Input: dimensioned drawing with shaded views. Units: mm. Origin: part minimum x, y, z. A direction names the side the tool comes from. Round coordinates to 2 decimals unless told otherwise and drop trailing zeros. Order: outer loops, then holes, each group sorted by start corner. A loop starts at its lowest first (then second) coordinate and runs counter-clockwise, first axis right, second up. Notation, with made-up numbers: M 75.5,74 L 80.5,74 A17 ccw 80.5,100 Z; hole C -10,42 d1. An arc over 180 degrees is marked long. Use one line per item in the form item = value. Start each with the question number.
Q1. Section A-A (y = 8). Return the cut outline in (x, z).
Q2. Contact query for flat-ended pins moving along their axis: pin 1 (8 mm diameter, centred on x = 2.5, y = 24, fed in from -Z); pin 2 (11 mm diameter, centred on y = 53, z = 24, fed in from +X); pin 3 (1 mm diameter, centred on x = 18.5, y = 42.5, fed in from +Z). Output: stop coordinate, or through.
Q3. Section D-D (y = 50). Return the cut outline in (x, z).
Q4. Material intervals for probe 1 along Y at (x, z) = (4.5, 20); probe 2 along Z at (x, y) = (14.25, 7.5), sorted ascending.
Q5. Reachability of the marked faces 1 and 2 from +Z, -Z, +X, -X, +Y, -Y: full face, straight path, thin tool, end or side. Return the list, or none.
Q6. Section B-B (x = 2.5). Return the cut outline in (y, z).
Q7. Section C-C (z = 24.5). Return the cut outline in (x, y), plus the area to 3 significant figures.
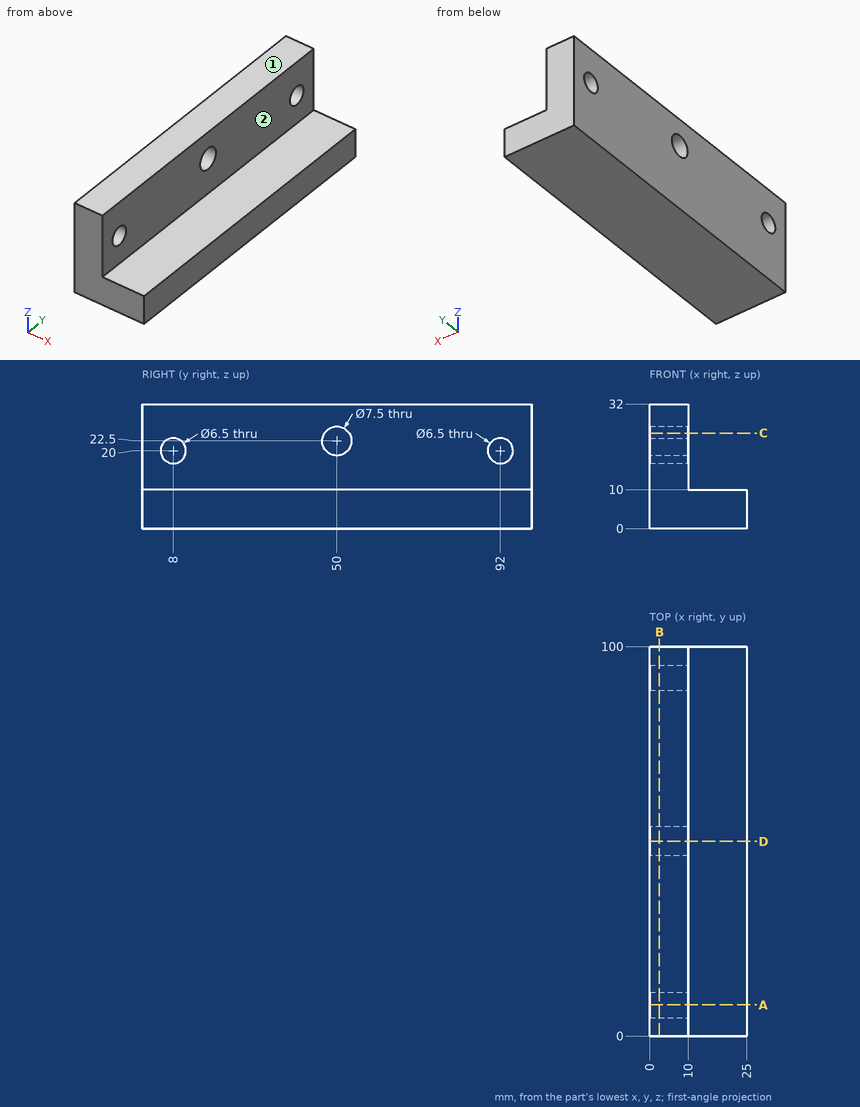
Results list:
q1.outline = M 0,0 L 25,0 L 25,10 L 10,10 L 10,16.75 L 0,16.75 Z; M 0,23.25 L 10,23.25 L 10,32 L 0,32 Z
q2.pin_1 = 0
q2.pin_2 = 10
q2.pin_3 = 10
q3.outline = M 0,0 L 25,0 L 25,10 L 10,10 L 10,18.75 L 0,18.75 Z; M 0,26.25 L 10,26.25 L 10,32 L 0,32 Z
q4.probe_1 = 0 to 4.75, 11.25 to 47.2, 52.8 to 88.75, 95.25 to 100
q4.probe_2 = 0 to 10
q5.face_1 = +Z, +X, -X, +Y, -Y
q5.face_2 = +Z, +X, +Y, -Y
q6.outline = M 0,0 L 100,0 L 100,32 L 0,32 Z; hole C 8,20 d6.5; hole C 50,22.5 d7.5; hole C 92,20 d6.5
q7.outline = M 0,0 L 10,0 L 10,46.83 L 0,46.83 Z; M 0,53.17 L 10,53.17 L 10,100 L 0,100 Z
q7.area = 937 mm2
